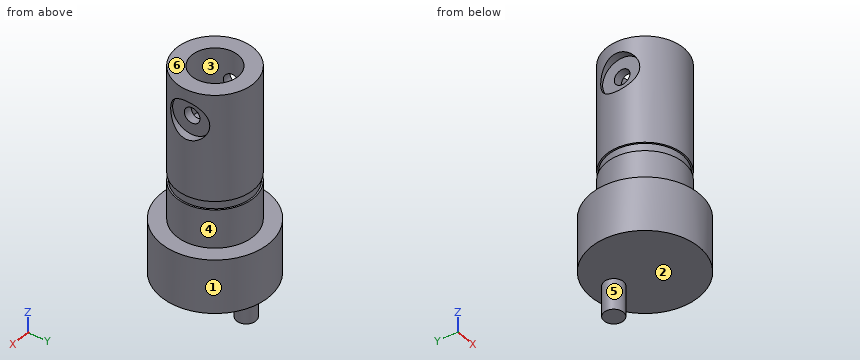
```python
from build123d import *

# Parameters (mm, degrees)
SKETCH1_R           = 7
BOSS_EXTRUDE1_DEPTH = 7
SKETCH2_R           = 5
BOSS_EXTRUDE2_DEPTH = 20
SKETCH3_R           = 6
SKETCH3_R_2         = 4.8
CUT_EXTRUDE1_DEPTH  = 1.1
SKETCH4_R           = 1.25
BOSS_EXTRUDE3_DEPTH = 4
SKETCH5_R           = 1
CUT_EXTRUDE2_DEPTH  = 13
SKETCH6_R           = 2.5
CUT_EXTRUDE3_DEPTH  = 1
SKETCH7_R           = 3
CUT_EXTRUDE4_DEPTH  = 8


with BuildPart() as part:
    # Sketch1 → Boss-Extrude1 (new body)
    with BuildSketch(Plane.XY):
        Circle(SKETCH1_R)
    extrude(amount=-BOSS_EXTRUDE1_DEPTH)

    # Sketch2 → Boss-Extrude2 (add)
    with BuildSketch(Plane.XY):
        Circle(SKETCH2_R)
    extrude(amount=BOSS_EXTRUDE2_DEPTH)

    # Sketch3 → Cut-Extrude1 (cut)
    with BuildSketch(Plane.XY.offset(5)):
        Circle(SKETCH3_R)
        Circle(SKETCH3_R_2, mode=Mode.SUBTRACT)
    extrude(amount=CUT_EXTRUDE1_DEPTH, mode=Mode.SUBTRACT)

    # Sketch4 → Boss-Extrude3 (add)
    with BuildSketch(Plane(origin=(0, 0, -7), x_dir=(-1, 0, 0), z_dir=(0, 0, -1))):
        with Locations((0, 4)):
            Circle(SKETCH4_R)
    extrude(amount=BOSS_EXTRUDE3_DEPTH)

    # Sketch5 → Cut-Extrude2 (cut, through all)
    with BuildSketch(Plane(origin=(5, 0, 0), x_dir=(0, 0, -1), z_dir=(1, 0, 0))):
        with Locations((-16, 0)):
            Circle(SKETCH5_R)
    extrude(amount=-CUT_EXTRUDE2_DEPTH, mode=Mode.SUBTRACT)

    # Sketch6 → Cut-Extrude3 (cut)
    with BuildSketch(Plane(origin=(5, 0, 0), x_dir=(0, 0, -1), z_dir=(1, 0, 0))):
        with Locations((-16, 0)):
            Circle(SKETCH6_R)
    cut_extrude3 = extrude(amount=-CUT_EXTRUDE3_DEPTH, mode=Mode.SUBTRACT)

    # Mirror1: Cut-Extrude3 across plane
    add(cut_extrude3.mirror(Plane(origin=(0, 0, 0), x_dir=(0, 0, 1), z_dir=(1, 0, 0))), mode=Mode.SUBTRACT)

    # Sketch7 → Cut-Extrude4 (cut)
    with BuildSketch(Plane.XY.offset(20)):
        Circle(SKETCH7_R)
    extrude(amount=-CUT_EXTRUDE4_DEPTH, mode=Mode.SUBTRACT)


solid = part.part
```
Part model, mm, in its own coordinate system. Face numbers are marked on the shaded views. A direction names the side the tool comes from. Give positions to 0.01 mm unless a question says otherwise; leave off trailing zeros. Write each loop counter-clockwise with the first axis right and the second up, starting at its lowest first coordinate (ties: lowest second). Pieces come first, ordered by that corner, then holes. Notation, with made-up numbers: M 27,-33.75 L 50,-33.75 A11 ccw 50,-23.75 Z; hole C -12,67.25 d2. An arc over 180 degrees is marked long. Use CSV: the item, a comma, the result in double quotes.
Item 1: Slice it at C-C on y = 4. Write the cut outline in (x, z), plus the area to 3 significant figures.
Taken from the geometry:
outline,"M -5.74,-7 L -1.25,-7 L -1.25,-11 L 1.25,-11 L 1.25,-7 L 5.74,-7 L 5.74,0 L 3,0 L 3,5 L 2.65,5 L 2.65,6.1 L 3,6.1 L 3,20 L -3,20 L -3,6.1 L -2.65,6.1 L -2.65,5 L -3,5 L -3,0 L -5.74,0 Z"
area,"210 mm²"
Item 2: Pin check, flat tips, straight feed: P1, Ø2.5, axis at y = -0.5, z = 16.5, coming from the -X side; P2, Ø1.6, axis at y = 0, z = 16, coming from the -X side; P3, Ø1, axis at y = -1.5, z = 5, coming from the -X side; P4, Ø1, axis at y = 5, z = 14, coming from the -X side. Stop position of each tip, or through.
Taken from the geometry:
P1,"stops at x = -4"
P2,"passes through"
P3,"stops at x = -4.9"
P4,"stops at x = -2.18"
Item 3: Drill centre lines: probe 1 along Y at (x, z) = (0, 17); probe 2 along Z at (x, y) = (-3.75, -3.25); probe 3 along X at (y, z) = (-3, 10.5). Where is each one in solid material? Low to high.
Taken from the geometry:
probe 1,"y = -5 to -3, 3 to 5"
probe 2,"z = -7 to 5, 6.1 to 20"
probe 3,"x = -4 to 4"
Item 4: Slice it at B-B on z = 16. Write the cut outline in (x, y), plus the area to 3 significant figures.
Taken from the geometry:
outline,"M -4.33,-2.5 A5 ccw 4.33,-2.5 L 4,-2.5 L 4,-1 L 2.83,-1 A3 cw -2.83,-1 L -4,-1 L -4,-2.5 Z; M -4.33,2.5 L -4,2.5 L -4,1 L -2.83,1 A3 cw 2.83,1 L 4,1 L 4,2.5 L 4.33,2.5 A5 ccw Z"
area,"38.2 mm²"
Item 5: Pull direction X, two halves, no side cores. Call the marked faces 1, 2 and 3: +X half, -X half, draft (parallel to the pull), parting line (faces both ways), or undercut.
Taken from the geometry:
face 1,"parting line"
face 2,"draft"
face 3,"undercut"
Item 6: Slice it at A-A on x = 0. Write the cut outline in (y, z), plus the area to 3 significant figures.
Taken from the geometry:
outline,"M -7,-7 L 2.75,-7 L 2.75,-11 L 5.25,-11 L 5.25,-7 L 7,-7 L 7,0 L 5,0 L 5,5 L 4.8,5 L 4.8,6.1 L 5,6.1 L 5,20 L 3,20 L 3,12 L -3,12 L -3,20 L -5,20 L -5,6.1 L -4.8,6.1 L -4.8,5 L -5,5 L -5,0 L -7,0 Z"
area,"260 mm²"
Item 7: Which spindle directions (+Z, -Z, +X, -X, +Y, -Y) get a long thin tool onto all of the face, cutting with end or side? Do the marked faces 4, 5 and 6. Say none if no direction does.
Taken from the geometry:
face 4,"+Z"
face 5,"-Z"
face 6,"+Z, +X, -X, +Y, -Y"
Item 8: Slice it at D-D on y = 0. State how many separate pieces and enclosed holes the cut face has, plus the area to 3 significant figures.
Taken from the geometry:
separate pieces,"3"
enclosed holes,"0"
area,"236 mm²"
